Read the model definition and answer for the solid it produces. Units are mm, in the model's axes. A direction names the side the tool comes from. Coordinates: 2 decimals unless noted, no trailing zeros. Loops run counter-clockwise (first coordinate to the right, second up) from the corner with the lowest first, then second, coordinate; pieces in that order, holes last.
Q1. Flat-ended cylindrical pins translate along their axes: P1, Ø1.5, axis at x = 5, y = -16.5, coming from the +Z side; P2, Ø1, axis at x = 4, y = -3.5, coming from the +Z side; P3, Ø3, axis at y = -7.5, z = 6.5, coming from the -X side. Find the tip coordinate at first contact, or state that the pin passes through.
Q2. Section A-A (x = 18) is taken. Give the vertices of the cut face in (y, z).
Q3. Straight lines are drawn through the part: line 1 (Y direction, x = 18, z = -1.6); line 2 (Z direction, x = 1.4, y = -6); line 3 (X direction, y = -0.75, z = 8). For each, find the intervals that lie inside material, in ascending order.
Q4. The mould has two halves that part along X. Classify faces 1 (the face through (-4.526, 7.352, -1.479)), 2 (the face through (6, -21, -1)), 3 (the face through (0, -7.4, 4.6)): pulls with the +X half, pulls with the -X half, needs draft (parallel to the pull), parting line crosses it, or undercut.
Q5. Section B-B (y = -18) is taken. Give the vertices of the cut face in (x, z).
Q6. Which of the six approach directions +Z, -Z, +X, -X, +Y, -Y give full straight-line access (tool end or side, diameter ignored) to faces 4 (the face through (6, -6, 2.366)), 5 (the face through (6, 9, -1)), 6 (the face through (6, -12, 1))?
Q7. Section D-D (z = 8) is taken. Give the vertices of the cut face in (x, y), then the cut area to 3 significant figures.
Q8. Section C-C (z = 3.5) is taken. Give the vertices of the cut face in (x, y), then the cut area to 3 significant figures.
from build123d import *

# Parameters (mm, degrees)
ESQUISSE1_W             = 12
ESQUISSE1_H             = 12
BOSS_EXTRU_1_DEPTH      = 12
ESQUISSE2_W             = 6
ESQUISSE2_H             = 9.63415441
ENL_V_MAT_EXTRU_1_DEPTH = 21.784609691
ESQUISSE3_R             = 2.5
ENL_V_MAT_EXTRU_2_DEPTH = 21.784609691
ESQUISSE4_W             = 30
ESQUISSE4_H             = 30
ESQUISSE4_R             = 2
BOSS_EXTRU_2_DEPTH      = 3


with BuildPart() as part:
    # Esquisse1 → Boss.-Extru.1 (new body)
    with BuildSketch(Plane.XY):
        with Locations((6, -6)):
            Rectangle(ESQUISSE1_W, ESQUISSE1_H)
    extrude(amount=BOSS_EXTRU_1_DEPTH)

    # Esquisse2 → Enlèv. mat.-Extru.1 (cut, through all)
    with BuildSketch(Plane(origin=(0, 0, 0), x_dir=(1, 0, 0), z_dir=(0, 1, 0))):
        with Locations((6, -7.182922795)):
            Rectangle(ESQUISSE2_W, ESQUISSE2_H)
    extrude(amount=-ENL_V_MAT_EXTRU_1_DEPTH, mode=Mode.SUBTRACT)

    # Esquisse3 → Enlèv. mat.-Extru.2 (cut, through all)
    with BuildSketch(Plane.ZY):
        with Locations(Location((7, -6, 0), (0, 0, 270))):
            Circle(ESQUISSE3_R)
        with BuildLine():
            Line((12, -12), (9, -12))
            ThreePointArc((9, -12), (10.960425347, -10.960425347), (12, -9))
            Line((12, -9), (12, -12))
        make_face()
        with BuildLine():
            Line((12, 0), (12, -3))
            ThreePointArc((12, -3), (11.019761374, -0.980238626), (9, 0))
            Line((9, 0), (12, 0))
        make_face()
    extrude(amount=-ENL_V_MAT_EXTRU_2_DEPTH, mode=Mode.SUBTRACT)

    # Esquisse4 → Boss.-Extru.2 (add)
    with BuildSketch(Plane(origin=(0, 0, 0), x_dir=(-1, 0, 0), z_dir=(0, 0, -1))):
        with Locations((-6, -6)):
            Rectangle(ESQUISSE4_W, ESQUISSE4_H)
        with Locations((-18, 6)):
            Circle(ESQUISSE4_R, mode=Mode.SUBTRACT)
        with Locations((6, 6)):
            Circle(ESQUISSE4_R, mode=Mode.SUBTRACT)
        with Locations((-18, -18)):
            Circle(ESQUISSE4_R, mode=Mode.SUBTRACT)
        with Locations((6, -18)):
            Circle(ESQUISSE4_R, mode=Mode.SUBTRACT)
    extrude(amount=BOSS_EXTRU_2_DEPTH)


solid = part.part
Numbers:
1. P1: stops at z = 0
1. P2: stops at z = 2.37
1. P3: stops at x = 0
2. outline: (-21, -3) - (-20, -3) - (-20, 0) - (-21, 0) - close; (-16, -3) - (4, -3) - (4, 0) - (-16, 0) - close; (8, -3) - (9, -3) - (9, 0) - (8, 0) - close
3. line 1: y = -21 to -20, -16 to 4, 8 to 9
3. line 2: z = -3 to 4.5, 9.5 to 12
3. line 3: x = 0 to 3, 9 to 12
4. face 1: undercut
4. face 2: needs draft
4. face 3: pulls with the -X half
5. outline: (-9, -3) - (-8, -3) - (-8, 0) - (-9, 0) - close; (-4, -3) - (16, -3) - (16, 0) - (-4, 0) - close; (20, -3) - (21, -3) - (21, 0) - (20, 0) - close
6. face 4: +Z, +Y, -Y
6. face 5: +Z, -Z, +X, -X, +Y
6. face 6: +Z, +X, -X, -Y
7. outline: (0, -12) - (3, -12) - (3, -8.29) - (0, -8.29) - close; (0, -3.71) - (3, -3.71) - (3, 0) - (0, 0) - close; (9, -12) - (12, -12) - (12, -8.29) - (9, -8.29) - close; (9, -3.71) - (12, -3.71) - (12, 0) - (9, 0) - close
7. area: 44.5 mm2
8. outline: (0, -12) - (3, -12) - (3, 0) - (0, 0) - close; (9, -12) - (12, -12) - (12, 0) - (9, 0) - close
8. area: 72.0 mm2
